from build123d import *

# Parameters (mm, degrees)
F0_W     = 20
F0_H     = 40
F1_DEPTH = 4
F2_W     = 9
F2_H     = 20
F2_W_2   = 20
F2_H_2   = 9
F3_DEPTH = 1
F4_SIZE  = 0.99999
F5_R     = 2.75
F6_DEPTH = 5.001
F7_SIZE  = 2


# Not quite as in the source:
# - a fillet or chamfer is up to 0.001 mm smaller than in the source, because OpenCascade refuses the exact size


with BuildPart() as f1:
    # F0 (on Top) → F1 (new body)
    with BuildSketch(Plane.XY):
        with Locations((10, 20)):
            Rectangle(F0_W, F0_H)
    extrude(amount=F1_DEPTH)

    # F2 (on face) → F3 (join)
    with BuildSketch(Plane.XY.offset(4)):
        with Locations((10, 30)):
            Rectangle(F2_W, F2_H)
        with Locations((10, 10)):
            Rectangle(F2_W_2, F2_H_2)
    extrude(amount=F3_DEPTH)

    # F4 (size 1 in the source; OpenCascade refuses exactly that, so slightly less here)
    f4_edges = [f1.edges().sort_by_distance(p)[0] for p in [
        (10, 40, 5),
        (5.5, 30, 5),
        (10, 20, 5),
        (14.5, 30, 5),
        (10, 14.5, 5),
        (0, 10, 5),
        (10, 5.5, 5),
        (20, 10, 5),
    ]]
    chamfer(f4_edges, length=F4_SIZE)

    # F5 (on face) → F6 (cut, through all)
    with BuildSketch(Plane.XY.offset(5)):
        with Locations((10, 30)):
            Circle(F5_R)
        with Locations((10, 10)):
            Circle(F5_R)
    extrude(amount=-F6_DEPTH, mode=Mode.SUBTRACT)

    # F7
    f7_edges = [f1.edges().sort_by_distance(p)[0] for p in [
        (0, 20, 0),
        (10, 0, 0),
        (20, 20, 0),
        (10, 40, 0),
    ]]
    chamfer(f7_edges, length=F7_SIZE)


solid = f1.part
Read the model definition and answer for the solid it produces. Units are mm, in the model's axes. A direction names the side the tool comes from. Round coordinates to 2 decimals unless told otherwise and drop trailing zeros. Write each loop counter-clockwise with the first axis right and the second up, starting at its lowest first coordinate (ties: lowest second). Pieces come first, ordered by that corner, then holes. Notation, with made-up numbers: (87.25, 18.25) - (126.25, 18.25) arc R7 cw to (126.25, 24.25) - close; hole circle Ø7 at (-13, -28). An arc over 180 degrees is marked (long way). Use a Markdown table: item, result.
(1) The mould has two halves that part along Y. Classify faces 5 (the flat face through (10, 20, 0)), 6 (the cylindrical face through (11.48, 32.32, 2.54)), 7 (the flat face through (9.9, 14, 4.5)), 8 (the flat face through (10, 39, 1)): released by +Y, released by -Y, zero draft, split by the parting line, or undercut.
Reported:
| item | result |
|---|---|
| face 5 | zero draft |
| face 6 | undercut |
| face 7 | undercut |
| face 8 | released by +Y |
(2) Straight lines are drawn through the part: line 1 along Y through (x, z) = (10, 2.8); line 2 along Y through (x, z) = (8.75, 3.65); line 3 along Z through (x, y) = (15, 31). For each, find the intervals that lie inside material, in ascending order. Write a range as [from, to].
Reported:
| item | result |
|---|---|
| line 1 | [0, 7.25], [12.75, 27.25], [32.75, 40] |
| line 2 | [0, 7.55], [12.45, 27.55], [32.45, 40] |
| line 3 | [0, 4] |
(3) The part is cut by section C-C (z = 3.35). Write down the section's boundary in (x, y), then the cut area to 3 significant figures.
Reported:
| item | result |
|---|---|
| outline | (0, 0) - (20, 0) - (20, 40) - (0, 40) - close; hole circle Ø5.5 at (10, 10); hole circle Ø5.5 at (10, 30) |
| area | 752 mm2 |
(4) Each of these flat-tipped pins is pushed along its axis until it touches: pin 1 Ø4.5 at (x, y) = (10, 30) entering from -Z; pin 2 Ø4.5 at (x, y) = (15, 3) entering from +Z. Where does it stop, or does it pass through?
Reported:
| item | result |
|---|---|
| pin 1 | through |
| pin 2 | z = 4 |
(5) The part is cut by section A-A (x = 10). State how many separate pieces and enclosed holes the cut face has, then the cut area to 3 significant figures.
Reported:
| item | result |
|---|---|
| separate pieces | 3 |
| enclosed holes | 0 |
| area | 128 mm2 |
(6) The part is cut by section B-B (y = 10). Write down the section's boundary in (x, z), then the cut area to 3 significant figures.
Reported:
| item | result |
|---|---|
| outline | (0, 2) - (2, 0) - (7.25, 0) - (7.25, 5) - (1, 5) - (0, 4) - close; (12.75, 0) - (18, 0) - (20, 2) - (20, 4) - (19, 5) - (12.75, 5) - close |
| area | 67.5 mm2 |
(7) Which of the six approach directions +Z, -Z, +X, -X, +Y, -Y give full straight-line access (tool end or side, diameter ignored) to faces 1 (the flat face through (10, 3, 4)), 2 (the flat face through (5, 25, 4)), 3 (the flat face through (6, 29.9, 4.5)), 4 (the flat face through (9.9, 20.5, 4.5))?
Reported:
| item | result |
|---|---|
| face 1 | +Z, +X, -X, -Y |
| face 2 | +Z |
| face 3 | +Z, -X, +Y |
| face 4 | +Z, +X, -X |
